The model under review builds one solid part; all positions refer to its coordinate system, in mm. A direction names the side the tool comes from. Round coordinates to 2 decimals unless told otherwise and drop trailing zeros. Loops run counter-clockwise (first coordinate to the right, second up) from the corner with the lowest first, then second, coordinate; pieces in that order, holes last. Notation, with made-up numbers: M 66,-30 L 99,-30 A13 ccw 99,-23 Z; hole C -20,85 d1. An arc over 180 degrees is marked long. Answer as a JSON object with one key per item and string values. Group by question number.
Item 1: The part is to be moulded in two halves that separate along X. For faces 1 (the face through (20.393, 2.465, 4.845)), 2 (the face through (-6.461, 2.465, -13.162)), 3 (the face through (-11, 4, 9.3)), say which applies: +X half, -X half, draft (parallel to the pull), parting line (faces both ways), or undercut.
Item 2: Consider section D-D (x = 11). Give the boundary of the cut face in (y, z).
Item 3: To check wall thickness, follow line 1 (Z direction, x = 0, y = 1.7); line 2 (X direction, y = 0.55, z = 7); line 3 (X direction, y = 1.15, z = 6.5). State the ranges of each line that lie inside material, in increasing order.
Item 4: Consider section B-B (y = 1.9). Give the boundary of the cut face in (x, z), and give its area (3 significant figures).
Item 5: Consider section A-A (x = 0). Give the boundary of the cut face in (y, z).
Item 6: Insertion check: P1, Ø2.5, axis at y = 2.5, z = -18, coming from the -X side; P2, Ø1.2, axis at x = 0, y = 4, coming from the +Z side; P3, Ø1.7, axis at x = 1, z = -14.5, coming from the +Y side; P4, Ø1.9, axis at x = -11.26, z = 6.5, coming from the +Y side. Each pin has a flat end and moves straight along its axis. Give the tip position at first contact, or say it passes through.
Item 7: Tool access review of faces 4 (the face through (-13.695, 3.768, 7.88)), 5 (the face through (6, 2, -20)), 6 (the face through (8.113, 2.465, 12.175)): name each direction out of +Z, -Z, +X, -X, +Y, -Y from which nothing blocks a thin tool from reaching the whole face with its end or side.
Item 8: Consider section C-C (z = 15.5). Give the boundary of the cut face in (x, y), and give its area (3 significant figures).
```python
from build123d import *

# Parameters (mm, degrees)
SKETCH1_R           = 8.05
SKETCH1_R_2         = 1.6
BOSS_EXTRUDE1_DEPTH = 5
CUT_EXTRUDE1_DEPTH  = 2.5
CUT_EXTRUDE2_REACH  = 4.5
SKETCH4_R           = 1.6


with BuildPart() as part:
    # Sketch1 → Boss-Extrude1 (new body)
    with BuildSketch(Plane(origin=(0, 0, 0), x_dir=(1, 0, 0), z_dir=(0, 1, 0))):
        with BuildLine():
            Line((24.650635095, -7.303847577), (16.013526617, -2.317210672))
            ThreePointArc((16.013526617, -2.317210672), (14.614747196, -0.962208024), (14.021609361, 0.892732285))
            ThreePointArc((14.021609361, 0.892732285), (12.167656923, 7.025), (7.783933518, 11.696703766))
            ThreePointArc((7.783933518, 11.696703766), (6.474077005, 13.137846354), (6, 15.02672619))
            Line((6, 15.02672619), (6, 25))
            ThreePointArc((6, 25), (0, 31), (-6, 25))
            Line((-6, 25), (-6, 15.02672619))
            ThreePointArc((-6, 15.02672619), (-6.474077005, 13.137846354), (-7.783933518, 11.696703766))
            ThreePointArc((-7.783933518, 11.696703766), (-12.167656923, 7.025), (-14.021609361, 0.892732285))
            ThreePointArc((-14.021609361, 0.892732285), (-14.614747196, -0.962208024), (-16.013526617, -2.317210672))
            Line((-16.013526617, -2.317210672), (-24.650635095, -7.303847577))
            ThreePointArc((-24.650635095, -7.303847577), (-26.846787517, -15.5), (-18.650635095, -17.696152423))
            Line((-18.650635095, -17.696152423), (-10.013526617, -12.709515518))
            ThreePointArc((-10.013526617, -12.709515518), (-8.140670191, -12.17563833), (-6.237675843, -12.589436051))
            ThreePointArc((-6.237675843, -12.589436051), (0, -14.05), (6.237675843, -12.589436051))
            ThreePointArc((6.237675843, -12.589436051), (8.140670191, -12.17563833), (10.013526617, -12.709515518))
            Line((10.013526617, -12.709515518), (18.650635095, -17.696152423))
            ThreePointArc((18.650635095, -17.696152423), (26.846787517, -15.5), (24.650635095, -7.303847577))
        make_face()
        Circle(SKETCH1_R, mode=Mode.SUBTRACT)
        with Locations((0, 25)):
            Circle(SKETCH1_R_2, mode=Mode.SUBTRACT)
        with Locations((21.650635095, -12.5)):
            Circle(SKETCH1_R_2, mode=Mode.SUBTRACT)
        with Locations((-21.650635095, -12.5)):
            Circle(SKETCH1_R_2, mode=Mode.SUBTRACT)
    extrude(amount=BOSS_EXTRUDE1_DEPTH)

    # Sketch3 → Cut-Extrude1 (cut)
    with BuildSketch(Plane(origin=(0, 5, 0), x_dir=(1, 0, 0), z_dir=(0, 1, 0))):
        Polygon((1.616580754, 15.8), (-1.616580754, 15.8), (-3.233161507, 13), (-1.616580754, 10.2), (1.616580754, 10.2), (3.233161507, 13), align=None)
        Polygon((-8.025168742, -6.5), (-9.641749495, -3.7), (-12.874911003, -3.7), (-14.491491757, -6.5), (-12.874911003, -9.3), (-9.641749495, -9.3), align=None)
        Polygon((14.491491757, -6.5), (12.874911003, -3.7), (9.641749495, -3.7), (8.025168742, -6.5), (9.641749495, -9.3), (12.874911003, -9.3), align=None)
    extrude(amount=-CUT_EXTRUDE1_DEPTH, mode=Mode.SUBTRACT)

    # Sketch4 → Cut-Extrude2 (cut, up to next)
    with BuildSketch(Plane(origin=(0, 2.5, 0), x_dir=(1, 0, 0), z_dir=(0, 1, 0)), mode=Mode.PRIVATE) as cut_extrude2_sk1:
        with Locations((0, 13)):
            Circle(SKETCH4_R)
    cut_extrude2_tool1 = extrude(cut_extrude2_sk1.sketch, amount=-CUT_EXTRUDE2_REACH, mode=Mode.PRIVATE) & part.part
    add(cut_extrude2_tool1.solids().sort_by_distance((0, 2.5, -13))[0], mode=Mode.SUBTRACT)
    # Sketch4 → Cut-Extrude2 (cut, up to next)
    with BuildSketch(Plane(origin=(0, 2.5, 0), x_dir=(1, 0, 0), z_dir=(0, 1, 0)), mode=Mode.PRIVATE) as cut_extrude2_sk2:
        with Locations((11.258330249, -6.5)):
            Circle(SKETCH4_R)
    cut_extrude2_tool2 = extrude(cut_extrude2_sk2.sketch, amount=-CUT_EXTRUDE2_REACH, mode=Mode.PRIVATE) & part.part
    add(cut_extrude2_tool2.solids().sort_by_distance((11.25833, 2.5, 6.5))[0], mode=Mode.SUBTRACT)
    # Sketch4 → Cut-Extrude2 (cut, up to next)
    with BuildSketch(Plane(origin=(0, 2.5, 0), x_dir=(1, 0, 0), z_dir=(0, 1, 0)), mode=Mode.PRIVATE) as cut_extrude2_sk3:
        with Locations((-11.258330249, -6.5)):
            Circle(SKETCH4_R)
    cut_extrude2_tool3 = extrude(cut_extrude2_sk3.sketch, amount=-CUT_EXTRUDE2_REACH, mode=Mode.PRIVATE) & part.part
    add(cut_extrude2_tool3.solids().sort_by_distance((-11.25833, 2.5, 6.5))[0], mode=Mode.SUBTRACT)


solid = part.part
```
Geometry results:
{
 "1": {"face 1": "+X half", "face 2": "-X half", "face 3": "undercut"},
 "2": {"outline": "M 0,-8.74 L 5,-8.74 L 5,3.7 L 2.5,3.7 L 2.5,4.92 L 0,4.92 Z; M 0,8.08 L 2.5,8.08 L 2.5,9.3 L 5,9.3 L 5,13.28 L 0,13.28 Z"},
 "3": {"line 1": "z = -31 to -26.6, -23.4 to -14.6, -11.4 to -8.05, 8.05 to 14.05", "line 2": "x = -24.12 to -12.78, -9.74 to -3.98, 3.98 to 9.74, 12.78 to 24.12", "line 3": "x = -23.26 to -12.86, -9.66 to -4.75, 4.75 to 9.66, 12.86 to 23.26"},
 "4": {"outline": "M -24.65,7.3 L -16.01,2.32 A4 cw -14.02,-0.89 A14.05 ccw -7.78,-11.7 A4 cw -6,-15.03 L -6,-25 A6 ccw 6,-25 L 6,-15.03 A4 cw 7.78,-11.7 A14.05 ccw 14.02,-0.89 A4 cw 16.01,2.32 L 24.65,7.3 A6 ccw 18.65,17.7 L 10.01,12.71 A4 cw 6.24,12.59 A14.05 ccw -6.24,12.59 A4 cw -10.01,12.71 L -18.65,17.7 A6 ccw Z; hole C -21.65,12.5 d3.2; hole C -11.26,6.5 d3.2; hole C 0,0 d16.1; hole C 0,-25 d3.2; hole C 0,-13 d3.2; hole C 11.26,6.5 d3.2; hole C 21.65,12.5 d3.2", "area": "953 mm^2"},
 "5": {"outline": "M 0,-31 L 5,-31 L 5,-26.6 L 0,-26.6 Z; M 0,-23.4 L 5,-23.4 L 5,-15.8 L 2.5,-15.8 L 2.5,-14.6 L 0,-14.6 Z; M 0,-11.4 L 2.5,-11.4 L 2.5,-10.2 L 5,-10.2 L 5,-8.05 L 0,-8.05 Z; M 0,8.05 L 5,8.05 L 5,14.05 L 0,14.05 Z"},
 "6": {"P1": "stops at x = -6", "P2": "stops at z = 14.05", "P3": "stops at y = 2.5", "P4": "passes through"},
 "7": {"face 4": "+Y", "face 5": "-Z, +X, +Y, -Y", "face 6": "+Z, +Y, -Y"},
 "8": {"outline": "M -26.85,0 L -14.85,0 L -14.85,5 L -26.85,5 Z; M 14.85,0 L 26.85,0 L 26.85,5 L 14.85,5 Z", "area": "120 mm^2"}
}
